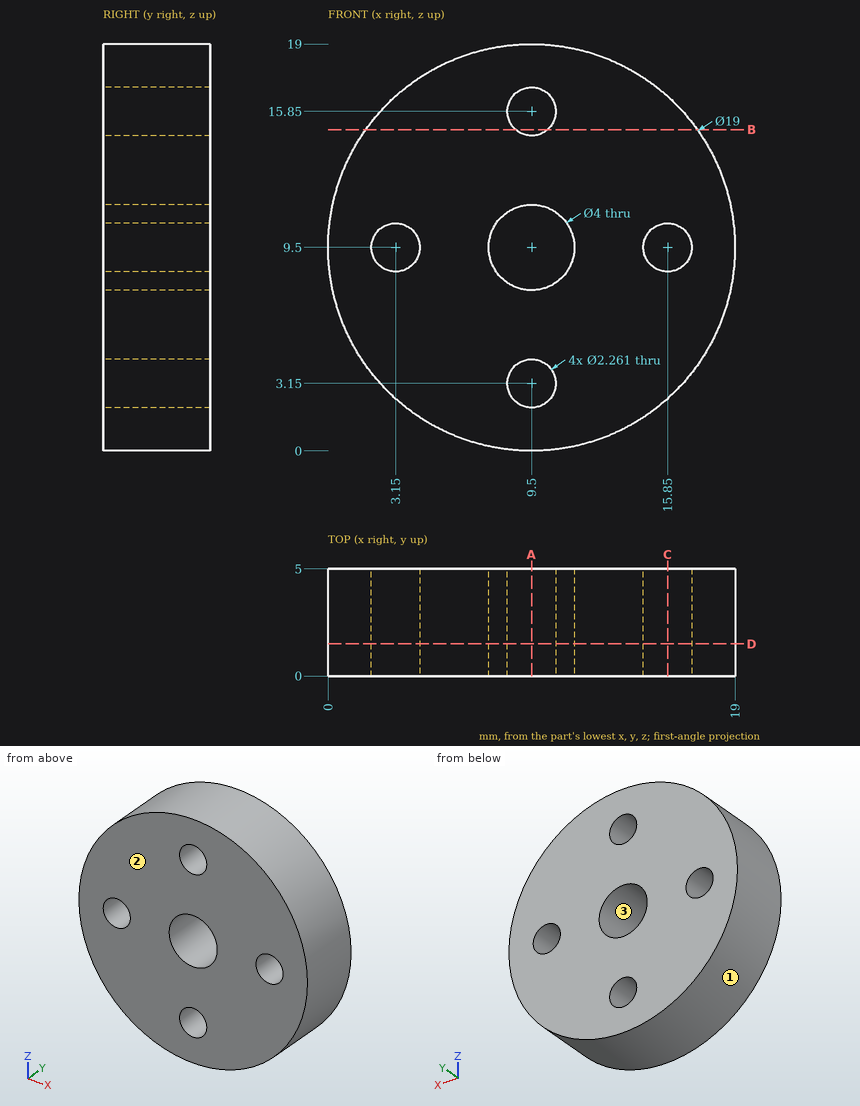
For this review, use the dimensioned drawing (mm, ordinates from the lowest corner) and the shaded views. Coordinates: 2 decimals unless noted, no trailing zeros. Loops run counter-clockwise (first coordinate to the right, second up) from the corner with the lowest first, then second, coordinate; pieces in that order, holes last.
1. For line 1 (Z direction, x = 9.5, y = 4); line 2 (Z direction, x = 8.25, y = 0.25); line 3 (Z direction, x = 15.85, y = 2.3) (1 decimal), list the stretches that pass through material, from the lowest coordinate up.
2. Add section B-B, the plane z = 15. Give the boundary of the cut face in (x, y) (1 decimal), then the cut area to 3 significant figures.
3. Add section A-A, the plane x = 9.5. Give the boundary of the cut face in (y, z).
4. Insertion check: P1, Ø1, axis at x = 7.5, y = 4, coming from the -Z side; P2, Ø1.4, axis at x = 15.85, z = 9.5, coming from the -Y side; P3, Ø1, axis at x = 14, y = 3, coming from the +Z side; P4, Ø1, axis at x = 4.5, y = 3, coming from the +Z side. Each pin has a flat end and moves straight along its axis. Give the tip position at first contact, or say it passes through.
5. Mouldability with a two-part tool opening along Z and no side actions: class the marked faces 1, 2 and 3 as +Z half, -Z half, draft (parallel to the pull), parting line (faces both ways), or undercut.
6. Add section D-D, the plane y = 1.5. Give the boundary of the cut face in (x, z).
7. Add section C-C, the plane x = 15.85. Give the boundary of the cut face in (y, z).
Result:
1. line 1: z = 0 to 2.02, 4.28 to 7.5, 11.5 to 14.72, 16.98 to 19
1. line 2: z = 0.08 to 7.94, 11.06 to 18.92
1. line 3: z = 2.4 to 8.4, 10.6 to 16.6
2. outline: (1.8, 0) - (8.8, 0) - (8.8, 5) - (1.8, 5) - close; (10.2, 0) - (17.2, 0) - (17.2, 5) - (10.2, 5) - close
2. area: 70.0 mm2
3. outline: (0, 0) - (5, 0) - (5, 2.02) - (0, 2.02) - close; (0, 4.28) - (5, 4.28) - (5, 7.5) - (0, 7.5) - close; (0, 11.5) - (5, 11.5) - (5, 14.72) - (0, 14.72) - close; (0, 16.98) - (5, 16.98) - (5, 19) - (0, 19) - close
4. P1: stops at z = 0.12
4. P2: passes through
4. P3: stops at z = 18.12
4. P4: stops at z = 17.87
5. face 1: parting line
5. face 2: draft
5. face 3: undercut
6. outline: circle Ø19 at (9.5, 9.5); hole circle Ø2.26 at (3.15, 9.5); hole circle Ø4 at (9.5, 9.5); hole circle Ø2.26 at (9.5, 3.15); hole circle Ø2.26 at (9.5, 15.85); hole circle Ø2.26 at (15.85, 9.5)
7. outline: (0, 2.43) - (5, 2.43) - (5, 8.37) - (0, 8.37) - close; (0, 10.63) - (5, 10.63) - (5, 16.57) - (0, 16.57) - close
